Can you work these out from the model? Positions are in its coordinate system, mm. A direction names the side the tool comes from. Give positions to 0.01 mm unless a question says otherwise; leave off trailing zeros. Loops run counter-clockwise (first coordinate to the right, second up) from the corner with the lowest first, then second, coordinate; pieces in that order, holes last. Notation, with made-up numbers: M 74,-32 L 104,-32 A17 ccw 104,-16 Z; hole C -3.75,83 d2. An arc over 180 degrees is marked long. Put each result on its own line as item: value. Start each with the question number.
1) Imagine slicing it at D-D (y = -9.4). Write out the boundary of the cut face in (x, z).
2) Imagine slicing it at B-B (y = 111). Write out the boundary of the cut face in (x, z), then the cut area to 3 significant figures.
3) Please list where these lines run through material, in increasing order: line 1 along Y through (x, z) = (-5, 14.25); line 2 along X through (y, z) = (-9, 54); line 3 along Y through (x, z) = (-0.6, 53). Write a range as from..to.
4) Imagine slicing it at C-C (z = 41). Write out the boundary of the cut face in (x, y).
5) For P1, Ø10, axis at x = -121.5, y = 65, coming from the +Z side; P2, Ø5, axis at y = 47, z = 27.5, coming from the -X side; P3, Ø2, axis at x = -62, y = -13.5, coming from the +Z side, each with a flat end and sliding along its axis, tell me the tip position at first contact or that it passes through.
6) If we mould it in two halves opening along X, with no side actions, what happens to faces 1 (the cylindrical face through (-7, 5, 14)), 2 (the flat face through (-4.2, -9, 30)), 3 (the flat face through (-73, 116, 1))? For each: +X half, -X half, draft (parallel to the pull), parting line (faces both ways), or undercut.
7) Imagine slicing it at A-A (z = 14.5). Write out the boundary of the cut face in (x, y).
8) For faces 4 (the flat face through (4, 42, 56)), 5 (the flat face through (-3, 3, 17.4)), 6 (the flat face through (-57, 111, 3.5)), 7 (the flat face through (-1, -9, 49.3)), 8 (the flat face through (-135, 42, 3.5)), which set-ups out of +Z, -Z, +X, -X, +Y, -Y let a thin tool reach every point of the face, with its end or its side?
from build123d import *

# Parameters (mm, degrees)
SKETCH_1_W      = 140
SKETCH_1_H      = 116
PAD_DEPTH       = 5
SKETCH_W        = 140
SKETCH_H        = 15
PAD001_DEPTH    = 5
SKETCH001_W     = 107
SKETCH001_H     = 2
PAD002_DEPTH    = 51
SKETCH002_W     = 15
SKETCH002_H     = 41
POCKET_DEPTH    = 2
SKETCH003_W     = 5
SKETCH003_H     = 131
PAD003_DEPTH    = 5
PAD004_DEPTH    = 51
SKETCH005_W     = 33
SKETCH005_H     = 2
PAD005_DEPTH    = 51
SKETCH006_R     = 3.6
PAD006_DEPTH    = 12.4
SKETCH007_R     = 2
POCKET001_DEPTH = 6.7
SKETCH008_W     = 122.1
SKETCH008_H     = 2.08
POCKET002_DEPTH = 11
SKETCH009_W     = 108.1
SKETCH009_H     = 2.08
POCKET003_DEPTH = 11
SKETCH010_W     = 7.2
SKETCH010_H     = 7.2
PAD007_DEPTH    = 51
SKETCH011_R     = 2
POCKET004_DEPTH = 6.7
PAD008_DEPTH    = 51
FILLET_R        = 2
CHAMFER_SIZE    = 2


with BuildPart() as part:
    # Sketch_1 → Pad (new body)
    with BuildSketch(Plane.XY):
        with Locations((-70, 58)):
            Rectangle(SKETCH_1_W, SKETCH_1_H)
    extrude(amount=PAD_DEPTH)

    # Sketch → Pad001 (join)
    with BuildSketch(Plane.XY):
        with Locations((-70, -7.5)):
            Rectangle(SKETCH_W, SKETCH_H)
    extrude(amount=PAD001_DEPTH)

    # Sketch001 (on Face8 of Pad001) → Pad002 (join)
    with BuildSketch(Plane.XY.offset(5)):
        with Locations((-53.5, -14)):
            Rectangle(SKETCH001_W, SKETCH001_H)
    extrude(amount=PAD002_DEPTH)

    # Sketch002 (on Face11 of Pad002) → Pocket (cut)
    with BuildSketch(Plane.XZ.offset(15)):
        with Locations((-23.5, 55.5)):
            Rectangle(SKETCH002_W, SKETCH002_H)
        with Locations((-43.5, 55.5)):
            Rectangle(SKETCH002_W, SKETCH002_H)
        with Locations((-63.5, 55.5)):
            Rectangle(SKETCH002_W, SKETCH002_H)
        with Locations((-83.5, 55.5)):
            Rectangle(SKETCH002_W, SKETCH002_H)
    extrude(amount=-POCKET_DEPTH, mode=Mode.SUBTRACT)

    # Sketch003 → Pad003 (join)
    with BuildSketch(Plane.XY):
        with Locations((2.5, 50.5)):
            Rectangle(SKETCH003_W, SKETCH003_H)
    extrude(amount=PAD003_DEPTH)

    # Sketch004 (on Face11 of Pad003) → Pad004 (join)
    with BuildSketch(Plane.XY.offset(5)):
        Polygon((5, 116), (3, 116), (3, -13), (0, -13), (0, -15), (5, -15), align=None)
    extrude(amount=PAD004_DEPTH)

    # Sketch005 (on Face8 of Pad004) → Pad005 (join)
    with BuildSketch(Plane.XY.offset(5)):
        with Locations((-123.5, -14)):
            Rectangle(SKETCH005_W, SKETCH005_H)
    extrude(amount=PAD005_DEPTH)

    # Sketch006 (on Face5 of Pad005) → Pad006 (join)
    with BuildSketch(Plane.XY.offset(5)):
        with Locations((-5, 5)):
            Circle(SKETCH006_R)
        with Locations((-5, 111)):
            Circle(SKETCH006_R)
    extrude(amount=PAD006_DEPTH)

    # Sketch007 (on Face25 of Pad006) → Pocket001 (cut)
    with BuildSketch(Plane.XY.offset(17.4)):
        with Locations((-5, 5)):
            Circle(SKETCH007_R)
        with Locations((-5, 111)):
            Circle(SKETCH007_R)
    extrude(amount=-POCKET001_DEPTH, mode=Mode.SUBTRACT)

    # Sketch008 (on Face3 of Pocket001) → Pocket002 (cut)
    with BuildSketch(Plane(origin=(0, 116, 0), x_dir=(-1, 0, 0), z_dir=(0, 1, 0))):
        with Locations((58, 2.46)):
            Rectangle(SKETCH008_W, SKETCH008_H)
    extrude(amount=-POCKET002_DEPTH, mode=Mode.SUBTRACT)

    # Sketch009 (on Face1 of Pocket002) → Pocket003 (cut)
    with BuildSketch(Plane(origin=(-140, 0, 0), x_dir=(0, -1, 0), z_dir=(-1, 0, 0))):
        with Locations((-41, 2.46)):
            Rectangle(SKETCH009_W, SKETCH009_H)
    extrude(amount=-POCKET003_DEPTH, mode=Mode.SUBTRACT)

    # Sketch010 (on Face16 of Pocket003) → Pad007 (join)
    with BuildSketch(Plane.XY.offset(5)):
        with Locations((-0.6, -9.4)):
            Rectangle(SKETCH010_W, SKETCH010_H)
    extrude(amount=PAD007_DEPTH)

    # Sketch011 (on Face41 of Pad007) → Pocket004 (cut)
    with BuildSketch(Plane.XY.offset(56)):
        with Locations((-0.6, -9.4)):
            Circle(SKETCH011_R)
    extrude(amount=-POCKET004_DEPTH, mode=Mode.SUBTRACT)

    # Sketch012 (on Face16 of Pocket004) → Pad008 (join)
    with BuildSketch(Plane.XY.offset(5)):
        Polygon((3, 116), (3, 114), (3, 113), (2, 114), (2, 117.5), (3, 117.5), align=None)
    extrude(amount=PAD008_DEPTH)

    # Fillet
    fillet_edges = [part.edges().sort_by_distance(p)[0] for p in [
        (-8.6, 5, 5),
        (-8.6, 111, 5),
    ]]
    fillet(fillet_edges, radius=FILLET_R)

    # Chamfer
    chamfer_edges = [part.edges().sort_by_distance(p)[0] for p in [
        (-91, -14, 35),
        (-71, -14, 35),
        (-76, -14, 35),
        (-56, -14, 35),
        (-51, -14, 35),
        (-36, -14, 35),
        (-31, -14, 35),
        (-16, -14, 35),
    ]]
    chamfer(chamfer_edges, length=CHAMFER_SIZE)


solid = part.part
Recorded:
1. outline: M -140,0 L 5,0 L 5,56 L 1.4,56 L 1.4,49.3 L -2.6,49.3 L -2.6,56 L -4.2,56 L -4.2,5 L -140,5 L -140,3.5 L -129,3.5 L -129,1.42 L -140,1.42 Z
2. outline: M -140,0 L 5,0 L 5,56 L 3,56 L 3,5 L 0.6,5 A2 cw -1.4,7 L -1.4,17.4 L -3,17.4 L -3,10.7 L -7,10.7 L -7,17.4 L -8.6,17.4 L -8.6,7 A2 cw -10.6,5 L -140,5 Z; hole M -119.05,1.42 L 3.05,1.42 L 3.05,3.5 L -119.05,3.5 Z
2. area: 637 mm²
3. line 1: -15..-13, 1.4..3, 7..8.6, 107.4..109, 113..114.6
3. line 2: -4.2..-2.56, 1.36..5
3. line 3: -15..-11.4, -7.4..-5.8
4. outline: M -140,-15 L -91,-15 L -91,-13 L -140,-13 Z; M -76,-15 L -71,-15 L -71,-13 L -76,-13 Z; M -56,-15 L -51,-15 L -51,-13 L -56,-13 Z; M -36,-15 L -31,-15 L -31,-13 L -36,-13 Z; M -16,-15 L 5,-15 L 5,116 L 3,116 L 3,117.5 L 2,117.5 L 2,114 L 3,113 L 3,-5.8 L -4.2,-5.8 L -4.2,-13 L -16,-13 Z
5. P1: z = 5
5. P2: x = 3
5. P3: z = 35
6. face 1: undercut
6. face 2: -X half
6. face 3: draft
7. outline: M -140,-15 L 5,-15 L 5,116 L 3,116 L 3,117.5 L 2,117.5 L 2,114 L 3,113 L 3,-5.8 L -4.2,-5.8 L -4.2,-13 L -140,-13 Z; C -5,5 d7.2; C -5,111 d7.2; hole C -5,5 d4; hole C -5,111 d4
8. face 4: +Z, +X, -X, +Y, -Y
8. face 5: +Z, -X, +Y
8. face 6: +Y
8. face 7: +Z
8. face 8: -X
